Verification items for the finished model (mm, model axes). Give positions to 0.01 mm unless a question says otherwise; leave off trailing zeros. Loops run counter-clockwise (first coordinate to the right, second up) from the corner with the lowest first, then second, coordinate; pieces in that order, holes last. Notation, with made-up numbers: (31.25, -19.5) - (63.25, -19.5) arc R20 ccw to (63.25, 6.5) - close; hole circle Ø11 at (34, -34). An arc over 180 degrees is marked (long way). One line per item, written item: value. Start each with the question number.
1. Gauge pin test, flat ends, axial feed: pin 1 (0.6 mm diameter, centred on x = 50.5, z = 1.5, fed in from -Y); pin 2 (3 mm diameter, centred on x = 62, y = 0, fed in from -Z); pin 3 (0.6 mm diameter, centred on x = -1.5, z = 1.5, fed in from -Y); pin 4 (1 mm diameter, centred on x = 52.5, z = 1.5, fed in from -Y). Record the tip position at first contact, or that the pin passes through.
2. Sectioned sample at C-C (y = 54). Record the cut outline in (x, z).
3. Scan lines: L1, parallel to Y at x = -31.5, z = 1.8; L2, parallel to Y at x = -62, z = 1.15; L3, parallel to X at y = 14.5, z = 1.6. Record each from-to range of solid material in increasing order. Write a range as [from, to].
4. Sectioned sample at D-D (x = -22). Record the cut outline in (y, z).
5. Sectioned sample at A-A (y = 12). Record the cut outline in (x, z), plus the area to 3 significant figures.
6. Sectioned sample at B-B (x = 54). Record the cut outline in (y, z).
from build123d import *

# Parameters (mm, degrees)
SKETCH1_W           = 90
SKETCH1_H           = 100
SKETCH1_H_2         = 22
SKETCH1_W_2         = 24
BOSS_EXTRUDE1_DEPTH = 2
CUT_EXTRUDE1_DEPTH  = 10
CUT_EXTRUDE2_DEPTH  = 10
SKETCH4_R           = 30
CUT_EXTRUDE3_DEPTH  = 10
CUT_EXTRUDE4_DEPTH  = 10
CUT_EXTRUDE5_DEPTH  = 10
BOSS_EXTRUDE3_START = -2
SKETCH8_R           = 30
SKETCH8_R_2         = 28
BOSS_EXTRUDE3_DEPTH = 2
SKETCH9_R           = 2
CUT_EXTRUDE6_DEPTH  = 10
SKETCH10_R          = 2
BOSS_EXTRUDE4_DEPTH = 2
SKETCH11_R          = 2
CUT_EXTRUDE7_DEPTH  = 10
SKETCH12_R          = 2
BOSS_EXTRUDE5_DEPTH = 2
SKETCH13_R          = 2
CUT_EXTRUDE8_DEPTH  = 5


with BuildPart() as part:
    # Sketch1 → Boss-Extrude1 (new body)
    with BuildSketch(Plane.XY):
        Rectangle(SKETCH1_W, SKETCH1_H)
        with Locations((0, 61)):
            Rectangle(SKETCH1_W, SKETCH1_H_2)
        with Locations((57, 0)):
            Rectangle(SKETCH1_W_2, SKETCH1_H)
        with BuildLine():
            Line((45, 50), (69, 50))
            ThreePointArc((69, 50), (61.278820596, 65.667804287), (45, 72))
            Line((45, 72), (45, 50))
        make_face()
        with BuildLine():
            ThreePointArc((45, -72), (61.83891888, -66.278820596), (69, -50))
            Line((69, -50), (45, -50))
            Line((45, -50), (45, -72))
        make_face()
        with Locations((0, -61)):
            Rectangle(SKETCH1_W, SKETCH1_H_2)
        with BuildLine():
            Line((-45, -72), (-45, -50))
            Line((-45, -50), (-69, -50))
            ThreePointArc((-69, -50), (-61.278820596, -65.667804287), (-45, -72))
        make_face()
        with Locations((-57, 0)):
            Rectangle(SKETCH1_W_2, SKETCH1_H)
        with BuildLine():
            Line((-69, 50), (-45, 50))
            Line((-45, 50), (-45, 72))
            ThreePointArc((-45, 72), (-61.83891888, 66.278820596), (-69, 50))
        make_face()
    extrude(amount=BOSS_EXTRUDE1_DEPTH)

    # Sketch2 → Cut-Extrude1 (cut)
    with BuildSketch(Plane.XY.offset(2)):
        with BuildLine():
            Line((-60.760739313, 25.787593916), (-64, 15.649215929))
            Line((-64, 15.649215929), (-64, 5))
            Line((-64, 5), (-43.724760028, 5))
            ThreePointArc((-43.724760028, 5), (-41.091915324, 15.757827722), (-35.856683042, 25.517698186))
            Line((-35.856683042, 25.517698186), (-56.217391304, 40.007560722))
            ThreePointArc((-56.217391304, 40.007560722), (-60.52773874, 33.126920216), (-64, 25.787593916))
            Line((-64, 25.787593916), (-60.760739313, 25.787593916))
        make_face()
        with BuildLine():
            Line((-64, -5), (-64, -25.787593916))
            ThreePointArc((-64, -25.787593916), (-60.52773874, -33.126920216), (-56.217391304, -40.007560722))
            Line((-56.217391304, -40.007560722), (-35.856683042, -25.517698186))
            ThreePointArc((-35.856683042, -25.517698186), (-41.091915324, -15.757827722), (-43.724760028, -5))
            Line((-43.724760028, -5), (-64, -5))
        make_face()
        with BuildLine():
            Line((-35.483097289, 48.383362913), (-26.026680798, 35.488963441))
            ThreePointArc((-26.026680798, 35.488963441), (-15.448259809, 41.209293956), (-3.716315379, 43.852521472))
            Line((-3.716315379, 43.852521472), (-5.066584601, 59.785698294))
            ThreePointArc((-5.066584601, 59.785698294), (-21.061160661, 56.182092446), (-35.483097289, 48.383362913))
        make_face()
        with BuildLine():
            ThreePointArc((64, 25.787593916), (60.52773874, 33.126920216), (56.217391304, 40.007560722))
            Line((56.217391304, 40.007560722), (35.856683042, 25.517698186))
            ThreePointArc((35.856683042, 25.517698186), (41.091915324, 15.757827722), (43.724760028, 5))
            Line((43.724760028, 5), (64, 5))
            Line((64, 5), (64, 25.787593916))
        make_face()
        with BuildLine():
            Line((-26.026680798, -35.488963441), (-35.483097289, -48.383362913))
            ThreePointArc((-35.483097289, -48.383362913), (-21.061160661, -56.182092446), (-5.066584601, -59.785698294))
            Line((-5.066584601, -59.785698294), (-3.716315379, -43.852521472))
            ThreePointArc((-3.716315379, -43.852521472), (-15.448259809, -41.209293956), (-26.026680798, -35.488963441))
        make_face()
        with BuildLine():
            ThreePointArc((56.217391304, -40.007560722), (60.52773874, -33.126920216), (64, -25.787593916))
            Line((64, -25.787593916), (64, -5))
            Line((64, -5), (43.724760028, -5))
            ThreePointArc((43.724760028, -5), (41.091915324, -15.757827722), (35.856683042, -25.517698186))
            Line((35.856683042, -25.517698186), (56.217391304, -40.007560722))
        make_face()
        with BuildLine():
            Line((27.916279909, 34.022580083), (38.059254795, 46.384190458))
            ThreePointArc((38.059254795, 46.384190458), (22.588514074, 55.585600941), (5.084745763, 59.784156434))
            Line((5.084745763, 59.784156434), (3.729636503, 43.851390526))
            ThreePointArc((3.729636503, 43.851390526), (16.568566174, 40.771770312), (27.916279909, 34.022580083))
        make_face()
        with BuildLine():
            Line((3.729636503, -43.851390526), (5.084745763, -59.784156434))
            ThreePointArc((5.084745763, -59.784156434), (22.588514074, -55.585600941), (38.059254795, -46.384190458))
            Line((38.059254795, -46.384190458), (27.916279909, -34.022580083))
            ThreePointArc((27.916279909, -34.022580083), (16.568566174, -40.771770312), (3.729636503, -43.851390526))
        make_face()
    extrude(amount=-CUT_EXTRUDE1_DEPTH, mode=Mode.SUBTRACT)

    # Sketch3 → Cut-Extrude2 (cut)
    with BuildSketch(Plane.XY.offset(2)):
        Polygon((-64, 25.787593916), (-64, 15.649215929), (-60.760739313, 25.787593916), align=None)
    extrude(amount=-CUT_EXTRUDE2_DEPTH, mode=Mode.SUBTRACT)

    # Sketch4 → Cut-Extrude3 (cut)
    with BuildSketch(Plane(origin=(0, 0, 0), x_dir=(-1, 0, 0), z_dir=(0, 0, -1))):
        Circle(SKETCH4_R)
    extrude(amount=-CUT_EXTRUDE3_DEPTH, mode=Mode.SUBTRACT)

    # Sketch6 → Cut-Extrude4 (cut)
    with BuildSketch(Plane.XY.offset(2)):
        Polygon((-35.856683042, -25.517698186), (-56.217391304, -40.007560722), (-50.280397209, -40.007560722), (-34.257403731, -27.258240508), align=None)
        Polygon((-50.280397209, 40.007560722), (-56.217391304, 40.007560722), (-35.856683042, 25.517698186), (-34.257403731, 27.258240508), align=None)
        Polygon((-50.280397209, -40.007560722), (-56.217391304, -40.007560722), (-53.993303971, -42.96187992), align=None)
        Polygon((-53.993303971, 42.96187992), (-56.217391304, 40.007560722), (-50.280397209, 40.007560722), align=None)
    extrude(amount=-CUT_EXTRUDE4_DEPTH, mode=Mode.SUBTRACT)

    # Sketch7 → Cut-Extrude5 (cut)
    with BuildSketch(Plane.XY.offset(2)):
        Polygon((-32.560271117, 27.267561972), (-24.823321267, 33.603144582), (-18.487738656, 25.866194731), (-26.224688507, 19.530612121), align=None)
        Polygon((27.827762823, 32.155388995), (19.915267174, 26.040455421), (26.030200748, 18.127959772), (33.942696396, 24.242893346), align=None)
        Polygon((33.988304577, -25.549058378), (27.336365779, -18.082351592), (19.869658993, -24.734290389), (26.521597791, -32.200997176), align=None)
        Polygon((-26.126682472, -33.612215797), (-18.478667441, -27.169555937), (-24.921327301, -19.521540905), (-32.569342333, -25.964200766), align=None)
    extrude(amount=-CUT_EXTRUDE5_DEPTH, mode=Mode.SUBTRACT)

    # Sketch8 → Boss-Extrude3 (add)
    with BuildSketch(Plane.XY.offset(2).offset(BOSS_EXTRUDE3_START)):
        Circle(SKETCH8_R)
        Circle(SKETCH8_R_2, mode=Mode.SUBTRACT)
    extrude(amount=BOSS_EXTRUDE3_DEPTH)

    # Sketch9 → Cut-Extrude6 (cut)
    with BuildSketch(Plane.XY.offset(2)):
        with Locations((13, 29.149963044)):
            Circle(SKETCH9_R)
        with Locations((-13, 29.149963044)):
            Circle(SKETCH9_R)
        with Locations((-22, 69)):
            Circle(SKETCH9_R)
        with Locations((22, 69)):
            Circle(SKETCH9_R)
        with Locations((62, -36.850036956)):
            Circle(SKETCH9_R)
        with Locations((-62, -36.850036956)):
            Circle(SKETCH9_R)
        with Locations((0, -36.850036956)):
            Circle(SKETCH9_R)
        with Locations((0, 65)):
            Circle(SKETCH9_R)
        with Locations((62, 0)):
            Circle(SKETCH9_R)
        with Locations((-62, 0)):
            Circle(SKETCH9_R)
        with Locations((0, -65)):
            Circle(SKETCH9_R)
        with Locations((-54, 54)):
            Circle(SKETCH9_R)
        with Locations((54, 54)):
            Circle(SKETCH9_R)
        with Locations((54, -54)):
            Circle(SKETCH9_R)
        with Locations((-54, -54)):
            Circle(SKETCH9_R)
        with Locations((-37.029437252, 37.029437252)):
            Circle(SKETCH9_R)
        with Locations((37.029437252, 37.029437252)):
            Circle(SKETCH9_R)
        with Locations((37.029437252, -37.029437252)):
            Circle(SKETCH9_R)
        with Locations((-37.029437252, -37.029437252)):
            Circle(SKETCH9_R)
    extrude(amount=-CUT_EXTRUDE6_DEPTH, mode=Mode.SUBTRACT)

    # Sketch10 → Boss-Extrude4 (add)
    with BuildSketch(Plane.XY.offset(2)):
        with Locations((62, -36.850036956)):
            Circle(SKETCH10_R)
        with Locations((-62, -36.850036956)):
            Circle(SKETCH10_R)
        with Locations((13, 29.149963044)):
            Circle(SKETCH10_R)
        with Locations((-13, 29.149963044)):
            Circle(SKETCH10_R)
        with Locations((0, -36.850036956)):
            Circle(SKETCH10_R)
    extrude(amount=-BOSS_EXTRUDE4_DEPTH)

    # Sketch11 → Cut-Extrude7 (cut)
    with BuildSketch(Plane.XY.offset(2)):
        with Locations((-62, -36)):
            Circle(SKETCH11_R)
        with Locations((62, -36)):
            Circle(SKETCH11_R)
    extrude(amount=-CUT_EXTRUDE7_DEPTH, mode=Mode.SUBTRACT)

    # Sketch12 → Boss-Extrude5 (add)
    with BuildSketch(Plane.XY.offset(2)):
        with Locations((62, -36)):
            Circle(SKETCH12_R)
        with Locations((-62, -36)):
            Circle(SKETCH12_R)
    extrude(amount=-BOSS_EXTRUDE5_DEPTH)

    # Sketch13 → Cut-Extrude8 (cut)
    with BuildSketch(Plane.XY.offset(2)):
        with Locations((62, -35)):
            Circle(SKETCH13_R)
        with Locations((-62, -35)):
            Circle(SKETCH13_R)
    extrude(amount=-CUT_EXTRUDE8_DEPTH, mode=Mode.SUBTRACT)


solid = part.part
Results are:
1. pin 1: stops at y = -71.84
1. pin 2: passes through
1. pin 3: stops at y = -72
1. pin 4: stops at y = -71.49
2. outline: (-68.63, 0) - (-56, 0) - (-56, 2) - (-68.63, 2) - close; (-52, 0) - (-26.15, 0) - (-26.15, 2) - (-52, 2) - close; (-4.58, 0) - (4.59, 0) - (4.59, 2) - (-4.58, 2) - close; (26.15, 0) - (52, 0) - (52, 2) - (26.15, 2) - close; (56, 0) - (68.31, 0) - (68.31, 2) - (56, 2) - close
3. L1: y = [-72, -51.07], [-42.95, -27.23], [-25.06, 25.97], [28.14, 42.95], [51.07, 72]
3. L2: y = [-64.98, -37], [-33, -30.28], [-5, -2], [2, 5], [30.28, 66.13]
3. L3: x = [-69, -64], [-41.55, -23.95], [23.95, 41.55], [64, 69]
4. outline: (-72, 0) - (-55.82, 0) - (-55.82, 2) - (-72, 2) - close; (-38.12, 0) - (-30.14, 0) - (-30.14, 2) - (-38.12, 2) - close; (-22.99, 0) - (-17.32, 0) - (-17.32, 2) - (-22.99, 2) - close; (17.32, 0) - (22.99, 0) - (22.99, 2) - (17.32, 2) - close; (30.16, 0) - (38.12, 0) - (38.12, 2) - (30.16, 2) - close; (55.82, 0) - (67, 0) - (67, 2) - (55.82, 2) - close; (71, 0) - (72, 0) - (72, 2) - (71, 2) - close
5. outline: (-69, 0) - (-64, 0) - (-64, 2) - (-69, 2) - close; (-42.34, 0) - (-25.3, 0) - (-25.3, 2) - (-42.34, 2) - close; (25.3, 0) - (42.34, 0) - (42.34, 2) - (25.3, 2) - close; (64, 0) - (69, 0) - (69, 2) - (64, 2) - close
5. area: 88.2 mm^2
6. outline: (-70.92, 0) - (-56, 0) - (-56, 2) - (-70.92, 2) - close; (-52, 0) - (-38.43, 0) - (-38.43, 2) - (-52, 2) - close; (-5, 0) - (5, 0) - (5, 2) - (-5, 2) - close; (38.43, 0) - (52, 0) - (52, 2) - (38.43, 2) - close; (56, 0) - (70.26, 0) - (70.26, 2) - (56, 2) - close
